Work out the finished part from the listing and answer in its coordinate system (mm). A direction names the side the tool comes from. Give positions to 0.01 mm unless a question says otherwise; leave off trailing zeros. Order: outer loops, then holes, each group sorted by start corner. A loop starts at its lowest first (then second) coordinate and runs counter-clockwise, first axis right, second up.
Autodesk Inventor part; units mm, degrees
ref_plane "YZ Plane" through (0, 0, 0) normal (1, 0, 0) x (0, 1, 0)
ref_plane "XZ Plane" through (0, 0, 0) normal (0, 1, 0) x (-1, 0, 0)
ref_plane "XY Plane" through (0, 0, 0) normal (0, 0, 1) x (1, 0, 0)
sketch "Sketch1" plane through (0, 0, 0) normal (0, 0, 1) x (1, 0, 0)
  line L0 (0, 0) -> (0, 17.78)
  line L1 (25.4, 17.78) -> (25.4, 0)
  arc A0 (25.4, 0) -> (0, 0) centre (12.7, -49.1869) ccw
  line L2 (0, 17.78) -> (3.175, 17.78)
  line L3 (3.175, 17.78) -> (12.7, 10.16)
  line L4 (12.7, 10.16) -> (22.225, 17.78)
  line L5 (22.225, 17.78) -> (25.4, 17.78)
  dimension "d4" = 17.78
  dimension "d5" = 25.4
  dimension "d6" = 101.6
  dimension "d7" = 3.175
  dimension "d8" = 7.62
extrude "Extrusion1" add sketch "Sketch1" along normal blind 25.4
chamfer "Chamfer1" distance 17.526 angle 45 2 edges at (23.8125, 17.78, 0) (1.5875, 17.78, 0)
chamfer "Chamfer2" distance 5.08 angle 45 2 edges at (25.4, 9.017, 8.763) (0, 9.017, 8.763)
fillet "Fillet1" radius 3.175 4 edges at (25.4, 8.89, 15.8202) (20.32, 8.6472, 8.3932) (5.08, 8.6472, 8.3932) (0, 8.89, 15.8202)
properties part number "RearMount" material "ABS Plastic"
1. Given P1, Ø8, axis at x = 10, z = 7.5, coming from the +Y side; P2, Ø1.5, axis at x = 21, y = 11, coming from the -Z side; P3, Ø6, axis at y = 14, z = 11.5, coming from the -X side, each flat-ended and moving along its own axis, determine where each tip first touches the part or whether it passes through.
Findings below:
P1: stops at y = 11.75
P2: stops at z = 10.71
P3: stops at x = 3.67
2. The part is cut by section B-B (x = 8.5). Write down the section's boundary in (y, z).
Findings below:
outline: (1.44, 1.19) - (13.52, 13.27) - (13.52, 25.4) - (1.44, 25.4) - close
3. The part is cut by section A-A (x = 20.5). Write down the section's boundary in (y, z), then the cut area to 3 significant figures.
Findings below:
outline: (1.01, 1.29) - (16.4, 16.68) - (16.4, 25.4) - (1.01, 25.4) - close
area: 253 mm2
4. Straight lines are drawn through the part: probe 1 along X at (y, z) = (14.75, 18.5); probe 2 along X at (y, z) = (10.75, 14.25); probe 3 along X at (y, z) = (3.75, 11). For each, find the intervals that lie inside material, in ascending order.
Findings below:
probe 1: x = 2.25 to 6.96, 18.44 to 23.15
probe 2: x = 2.43 to 11.96, 13.44 to 22.97
probe 3: x = 0.19 to 25.21
5. The mould has two halves that part along X. Classify faces 1 (the face through (12.52, 1.613, 13.003)), 2 (the face through (0, 4, 21)), 3 (the face through (2, 17.78, 23)): pulls with the +X half, pulls with the -X half, needs draft (parallel to the pull), parting line crosses it, or undercut.
Findings below:
face 1: undercut
face 2: pulls with the -X half
face 3: needs draft
6. Which of the six approach directions +Z, -Z, +X, -X, +Y, -Y give full straight-line access (tool end or side, diameter ignored) to faces 4 (the face through (16.34, 13.07, 19.27)), 5 (the face through (22.88, 9.18, 12.55))?
Findings below:
face 4: +Z, -Z, +Y
face 5: -Z, +X, +Y
